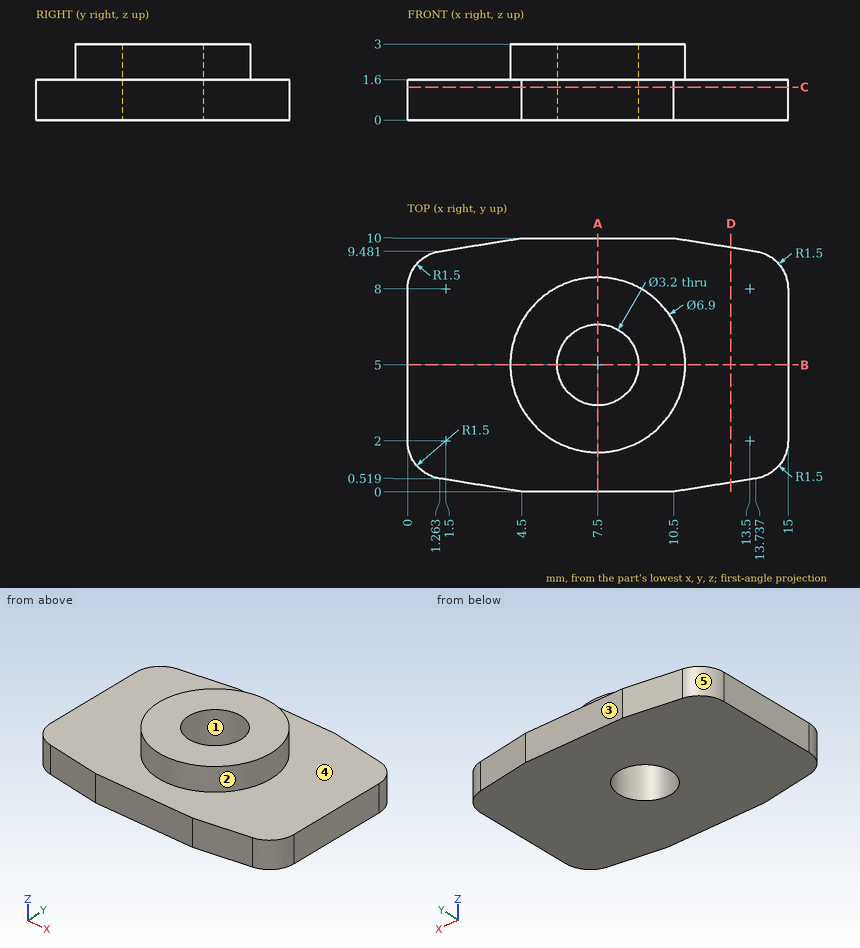
Geometry check sheet. Reference: drawing and pictorial views, mm from the part's lowest x, y, z. A direction names the side the tool comes from. Coordinates: 2 decimals unless noted, no trailing zeros. Loops run counter-clockwise (first coordinate to the right, second up) from the corner with the lowest first, then second, coordinate; pieces in that order, holes last. Notation, with made-up numbers: (41.5, 39.5) - (49.5, 39.5) arc R25 ccw to (49.5, 59.5) - close; hole circle Ø1 at (1.5, -13.5). An arc over 180 degrees is marked (long way). Return JSON: item names as keys, results as strings.
1. Section check C-C, the plane z = 1.3. Record the boundary of the cut face in (x, y).
Established:
{"outline": "(0, 2) arc R1.5 ccw to (1.26, 0.52) - (4.5, 0) - (10.5, 0) - (13.74, 0.52) arc R1.5 ccw to (15, 2) - (15, 8) arc R1.5 ccw to (13.74, 9.48) - (10.5, 10) - (4.5, 10) - (1.26, 9.48) arc R1.5 ccw to (0, 8) - close; hole circle Ø3.2 at (7.5, 5)"}
2. Section check A-A, the plane x = 7.5. Record the boundary of the cut face in (y, z).
Established:
{"outline": "(0, 0) - (3.4, 0) - (3.4, 3) - (1.55, 3) - (1.55, 1.6) - (0, 1.6) - close; (6.6, 0) - (10, 0) - (10, 1.6) - (8.45, 1.6) - (8.45, 3) - (6.6, 3) - close"}
3. Section check D-D, the plane x = 12.75. Record the boundary of the cut face in (y, z).
Established:
{"outline": "(0.36, 0) - (9.64, 0) - (9.64, 1.6) - (0.36, 1.6) - close"}
4. Section check B-B, the plane y = 5. Record the boundary of the cut face in (x, z).
Established:
{"outline": "(0, 0) - (5.9, 0) - (5.9, 3) - (4.05, 3) - (4.05, 1.6) - (0, 1.6) - close; (9.1, 0) - (15, 0) - (15, 1.6) - (10.95, 1.6) - (10.95, 3) - (9.1, 3) - close"}
5. Tool access check on the marked faces 4 and 5. Record the directions out of +Z, -Z, +X, -X, +Y, -Y that give a thin tool (end or side, any length) a straight path to the whole face; none if there is none.
Established:
{"face 4": "+Z", "face 5": "+Z, -Z, -X, +Y"}
6. Mould release check, pull along X, two halves, no side actions. Record for the marked faces 1, 2 and 3: +X half, -X half, draft (parallel to the pull), parting line (faces both ways), or undercut.
Established:
{"face 1": "undercut", "face 2": "parting line", "face 3": "draft"}
7. Go/stop test with flat-tipped pins: pin 1 (2 mm diameter, centred on x = 4, y = 4.5, fed in from +Z); pin 2 (3 mm diameter, centred on x = 13, y = 4, fed in from +Z). Record where each tip stops, or that it passes through.
Established:
{"pin 1": "stops at z = 3", "pin 2": "stops at z = 1.6"}
8. Thickness scan on L1, parallel to Y at x = 7.5, z = 0.8; L2, parallel to Y at x = 7.5, z = 2.2; L3, parallel to Z at x = 10.5, y = 8.5. Record the ranges inside material, lowest first.
Established:
{"L1": "y = 0 to 3.4, 6.6 to 10", "L2": "y = 1.55 to 3.4, 6.6 to 8.45", "L3": "z = 0 to 1.6"}
